Input: part model. Units: mm. Frame: model coordinates. Give positions to 0.01 mm unless a question says otherwise; leave off trailing zeros. Loops run counter-clockwise (first coordinate to the right, second up) from the corner with the lowest first, then second, coordinate; pieces in that order, holes last. Notation, with made-up numbers: (79, -20.75) - (94, -20.75) arc R35 cw to (94, 11.25) - close; hole circle Ø11 at (3.5, 49). An arc over 180 degrees is marked (long way). Answer as a JSON object with one key per item and string values. Group by question number.
(1) Section query A-A (y = -45). Return loops of the section in (x, z).
(2) Material intervals for L1, parallel to Y at x = 0.5, z = 3.4; L2, parallel to X at y = -44.5, z = 1.95; L3, parallel to X at y = -34, z = 3, sorted ascending.
(3) Section query D-D (z = 3.1). Count the separate pieces of the cut face and the enclosed holes in it, plus the area to 3 significant figures.
(4) Section query B-B (y = -14). Return loops of the section in (x, z).
(5) Section query C-C (x = -20). Return loops of the section in (y, z).
(6) Pin query (flat end, axial travel): P1, Ø2, axis at y = -44, z = 2, coming from the -X side. Return the tip coordinate at first contact, or that it passes through.
```python
from build123d import *

# Parameters (mm, degrees)
SCHIZZO1_R                   = 2.5
SCHIZZO1_R_2                 = 1.5
ESTRUSIONE_ESTRUSIONE1_DEPTH = 4
TAGLIO_ESTRUSIONE1_DEPTH     = 77.399732917
SCHIZZO3_R                   = 1.5
TAGLIO_ESTRUSIONE2_DEPTH     = 77.399732917
CROQUIS1_W                   = 9
CROQUIS1_H                   = 19.861523984
CORTAR_EXTRUIR1_DEPTH        = 10


with BuildPart() as part:
    # Schizzo1 → Estrusione-Estrusione1 (new body)
    with BuildSketch(Plane.XY):
        with BuildLine():
            Line((15, -50), (-35, -50))
            Line((-35, -50), (-35, -31.140095692))
            Line((-35, -31.140095692), (-57.627416998, -10.021990785))
            Line((-57.627416998, -10.021990785), (-57.627416998, 4.978009215))
            Line((-57.627416998, 4.978009215), (-27.627416998, 18.859904308))
            Line((-27.627416998, 18.859904308), (-27.627416998, 22.627416998))
            ThreePointArc((-27.627416998, 22.627416998), (-26.162950904, 26.162950904), (-22.627416998, 27.627416998))
            Line((-22.627416998, 27.627416998), (19.155603231, 27.627416998))
            ThreePointArc((19.155603231, 27.627416998), (35.964766047, 18.464946487), (37.372583002, -0.627378458))
            Line((37.372583002, -0.627378458), (15, -50))
        make_face()
        Circle(SCHIZZO1_R, mode=Mode.SUBTRACT)
        with Locations((-20, -45)):
            Circle(SCHIZZO1_R_2, mode=Mode.SUBTRACT)
        with Locations((0, -45)):
            Circle(SCHIZZO1_R_2, mode=Mode.SUBTRACT)
        with Locations((-22.627416998, 22.627416998)):
            Circle(SCHIZZO1_R_2, mode=Mode.SUBTRACT)
    extrude(amount=ESTRUSIONE_ESTRUSIONE1_DEPTH)

    # Schizzo2 → Taglio-Estrusione1 (cut, through all)
    with BuildSketch(Plane.XY.offset(4)):
        with BuildLine():
            Line((-27.856099407, -12.90456221), (-2.268412004, -1.050860115))
            ThreePointArc((-2.268412004, -1.050860115), (-1.050860115, 2.268412004), (2.268412004, 1.050860115))
            Line((2.268412004, 1.050860115), (9.073648015, 4.203440459))
            Line((9.073648015, 4.203440459), (4.870207556, 13.277088475))
            Line((4.870207556, 13.277088475), (-32.059539866, -3.830914194))
            Line((-32.059539866, -3.830914194), (-27.856099407, -12.90456221))
        make_face()
        with BuildLine():
            ThreePointArc((2.5, 0), (0.538038098, -2.441416598), (-2.268412004, -1.050860115))
            Line((-2.268412004, -1.050860115), (-27.856099407, -12.90456221))
            Line((-27.856099407, -12.90456221), (-23.652658948, -21.978210225))
            Line((-23.652658948, -21.978210225), (13.277088475, -4.870207556))
            Line((13.277088475, -4.870207556), (9.073648015, 4.203440459))
            Line((9.073648015, 4.203440459), (2.268412004, 1.050860115))
            ThreePointArc((2.268412004, 1.050860115), (2.441416598, 0.538038098), (2.5, 0))
        make_face()
    extrude(amount=-TAGLIO_ESTRUSIONE1_DEPTH, mode=Mode.SUBTRACT)

    # Schizzo3 → Taglio-Estrusione2 (cut, through all)
    with BuildSketch(Plane.XY.offset(4)):
        with Locations((10.601386992, 10.421640651)):
            Circle(SCHIZZO3_R)
        with Locations((14.804827451, 1.347992635)):
            Circle(SCHIZZO3_R)
        with Locations((-29.383838384, -19.122762401)):
            Circle(SCHIZZO3_R)
        with Locations((-33.587278843, -10.049114386)):
            Circle(SCHIZZO3_R)
    extrude(amount=-TAGLIO_ESTRUSIONE2_DEPTH, mode=Mode.SUBTRACT)

    # Croquis1 → Cortar-Extruir1 (cut)
    with BuildSketch(Plane(origin=(0, 0, 0), x_dir=(-1, 0, 0), z_dir=(0, 0, -1))):
        with Locations((-19.5, -40.069238008)):
            Rectangle(CROQUIS1_W, CROQUIS1_H)
    extrude(amount=-CORTAR_EXTRUIR1_DEPTH, mode=Mode.SUBTRACT)


solid = part.part
```
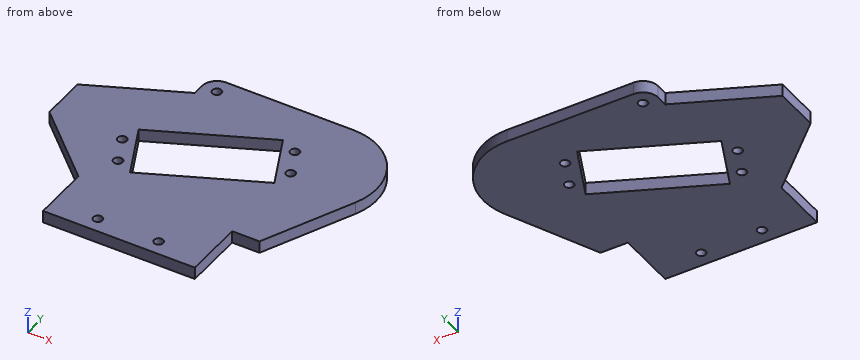
Recorded:
{
 "1": {"outline": "(-35, 0) - (-21.5, 0) - (-21.5, 4) - (-35, 4) - close; (-18.5, 0) - (-1.5, 0) - (-1.5, 4) - (-18.5, 4) - close; (1.5, 0) - (15, 0) - (15, 4) - (1.5, 4) - close"},
 "2": {"L1": "y = -50 to -46.41, -43.59 to -10.79, 11.25 to 27.63", "L2": "x = -35 to -21.41, -18.59 to -1.41, 1.41 to 15", "L3": "x = -35 to 15"},
 "3": {"separate pieces": "1", "enclosed holes": "8", "area": "4,690 mm^2"},
 "4": {"outline": "(-53.37, 0) - (-27.35, 0) - (-27.35, 4) - (-53.37, 4) - close; (-6.43, 0) - (31.31, 0) - (31.31, 4) - (-6.43, 4) - close"},
 "5": {"outline": "(-50, 0) - (-46.5, 0) - (-46.5, 4) - (-50, 4) - close; (-43.5, 0) - (-20.29, 0) - (-20.29, 4) - (-43.5, 4) - close; (1.76, 0) - (27.63, 0) - (27.63, 4) - (1.76, 4) - close"},
 "6": {"P1": "stops at x = -35"}
}
